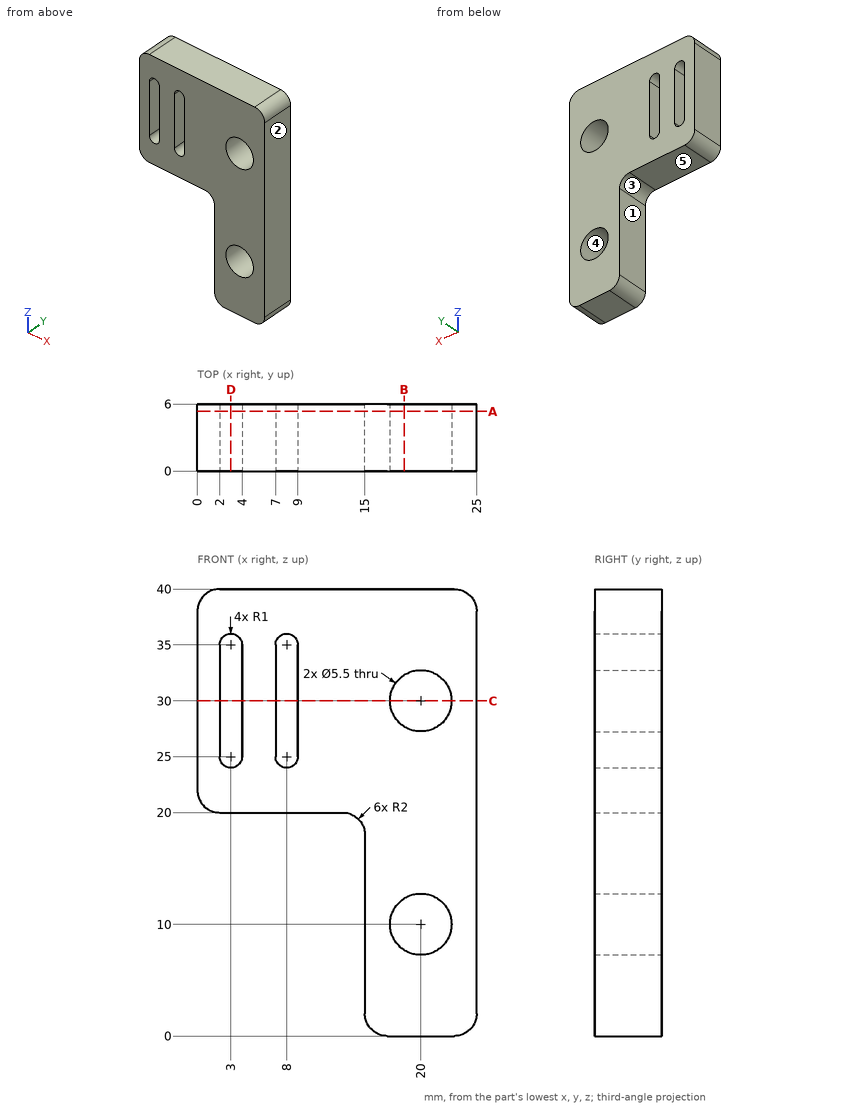
Answer from the drawing. Dimensions are ordinates in mm from the lowest x, y and z of the part. A direction names the side the tool comes from. Coordinates: 2 decimals unless noted, no trailing zeros. Write each loop counter-clockwise with the first axis right and the second up, starting at its lowest first coordinate (ties: lowest second). Pieces come first, ordered by that corner, then holes. Notation, with made-up numbers: (68, 42) - (125, 42) arc R12 ccw to (125, 65) - close; hole circle Ø6 at (6.25, 44.25). An arc over 180 degrees is marked (long way). Return JSON: item names as keys, results as strings. Group by question number.
Q1. The part is cut by section B-B on x = 18.5. Write down the section's boundary in (y, z).
Q2. For a pull along X with two mould halves and no side action, classify the marked faces 3, 4 and 5 as +X half, -X half, draft (parallel to the pull), parting line (faces both ways), or undercut.
Q3. The part is cut by section D-D on x = 3. Write down the section's boundary in (y, z), and give its area (3 significant figures).
Q4. Find the intervals of material crossed by line 1 along X through (y, z) = (1.75, 30); line 2 along X through (y, z) = (4.75, 33.5); line 3 along Z through (x, y) = (20, 3.6), in increasing order. Write a range as [from, to].
Q5. Which of the six approach directions +Z, -Z, +X, -X, +Y, -Y give full straight-line access (tool end or side, diameter ignored) to the marked faces 1 and 2?
Q6. The part is cut by section A-A on y = 5.35. Write down the section's boundary in (x, z).
Q7. Flat-ended cylindrical pins translate along their axes: pin 1 Ø3 at (x, y) = (5, 4) entering from -Z; pin 2 Ø3 at (y, z) = (3.5, 7.5) entering from -X. Find the tip coordinate at first contact, or state that the pin passes through.
Q8. The part is cut by section C-C on z = 30. Write down the section's boundary in (x, y).
Evaluation:
{
 "1": {"outline": "(0, 0) - (6, 0) - (6, 7.7) - (0, 7.7) - close; (0, 12.3) - (6, 12.3) - (6, 27.7) - (0, 27.7) - close; (0, 32.3) - (6, 32.3) - (6, 40) - (0, 40) - close"},
 "2": {"face 3": "-X half", "face 4": "undercut", "face 5": "draft"},
 "3": {"outline": "(0, 20) - (6, 20) - (6, 24) - (0, 24) - close; (0, 36) - (6, 36) - (6, 40) - (0, 40) - close", "area": "48.0 mm2"},
 "4": {"line 1": "x = [0, 2], [4, 7], [9, 17.25], [22.75, 25]", "line 2": "x = [0, 2], [4, 7], [9, 25]", "line 3": "z = [0, 7.25], [12.75, 27.25], [32.75, 40]"},
 "5": {"face 1": "-Z, -X, +Y, -Y", "face 2": "+Z, -Z, +X, +Y, -Y"},
 "6": {"outline": "(0, 22) arc R2 ccw to (2, 20) - (13, 20) arc R2 cw to (15, 18) - (15, 2) arc R2 ccw to (17, 0) - (23, 0) arc R2 ccw to (25, 2) - (25, 38) arc R2 ccw to (23, 40) - (2, 40) arc R2 ccw to (0, 38) - close; hole (2, 25) arc R1 ccw to (4, 25) - (4, 35) arc R1 ccw to (2, 35) - close; hole (7, 25) arc R1 ccw to (9, 25) - (9, 35) arc R1 ccw to (7, 35) - close; hole circle Ø5.5 at (20, 10); hole circle Ø5.5 at (20, 30)"},
 "7": {"pin 1": "stops at z = 20", "pin 2": "stops at x = 15"},
 "8": {"outline": "(0, 0) - (2, 0) - (2, 6) - (0, 6) - close; (4, 0) - (7, 0) - (7, 6) - (4, 6) - close; (9, 0) - (17.25, 0) - (17.25, 6) - (9, 6) - close; (22.75, 0) - (25, 0) - (25, 6) - (22.75, 6) - close"}
}
